```python
from build123d import *

# Parameters (mm, degrees)
BOSS_EXTRUDE1_DEPTH                = 25.4
FILLET1_R                          = 25.4
F_1_4_0_25_DIAMETER_SLOT1_DEPTH    = 25.4
F_1_16_0_0625_DIAMETER_HOLE1_D     = 1.5875
F_1_16_0_0625_DIAMETER_HOLE1_DEPTH = 12.7
F_1_16_0_0625_DIAMETER_HOLE1_TIP   = 0.476933116


# Read off the part's stored shape, not the designer's step: 1/4 (0.25) Diameter Slot1
with BuildPart() as part:
    # Sketch1 → Boss-Extrude1 (new body)
    with BuildSketch(Plane.XY):
        Polygon((-152.4, 0), (152.4, 0), (122.789463707, -63.5), (-122.789463707, -63.5), align=None)
    extrude(amount=BOSS_EXTRUDE1_DEPTH)

    # Fillet1
    fillet1_edges = [part.edges().sort_by_distance(p)[0] for p in [
        (122.789463707, -63.5, 12.7),
        (-122.789463707, -63.5, 12.7),
    ]]
    fillet(fillet1_edges, radius=FILLET1_R)

    # 1/4 (0.25) Diameter Slot1 outline → 1/4 (0.25) Diameter Slot1 (cut)
    with BuildSketch(Plane.XY):
        with BuildLine():
            Line((-92.075, -41.275), (92.075, -41.275))
            ThreePointArc((92.075, -41.275), (95.25, -38.1), (92.075, -34.925))
            Line((92.075, -34.925), (-92.075, -34.925))
            ThreePointArc((-92.075, -34.925), (-95.25, -38.1), (-92.075, -41.275))
        make_face()
    extrude(amount=F_1_4_0_25_DIAMETER_SLOT1_DEPTH, mode=Mode.SUBTRACT)

    # 1/16 (0.0625) Diameter Hole1
    with Locations(Plane(origin=(0, 0, 0), x_dir=(1, 0, 0), z_dir=(0, 1, 0))):
        with Locations((-101.6, -12.7), (-50.8, -12.7), (0, -12.7), (50.8, -12.7), (101.6, -12.7)):
            Hole(F_1_16_0_0625_DIAMETER_HOLE1_D / 2, depth=F_1_16_0_0625_DIAMETER_HOLE1_DEPTH)
            with Locations((0, 0, -(F_1_16_0_0625_DIAMETER_HOLE1_DEPTH + F_1_16_0_0625_DIAMETER_HOLE1_TIP / 2))):  # 118° drill point
                Cone(0, F_1_16_0_0625_DIAMETER_HOLE1_D / 2, F_1_16_0_0625_DIAMETER_HOLE1_TIP, mode=Mode.SUBTRACT)


solid = part.part
```
The listing builds one solid part. Answer for the finished solid, in the listing's coordinates (mm). A direction names the side the tool comes from. Coordinates: 2 decimals unless noted, no trailing zeros. Write each loop counter-clockwise with the first axis right and the second up, starting at its lowest first coordinate (ties: lowest second). Pieces come first, ordered by that corner, then holes. Notation, with made-up numbers: (26.5, 4) - (30.5, 4) arc R17 ccw to (30.5, 32) - close; hole circle Ø11 at (39, -23). An arc over 180 degrees is marked (long way). Return JSON: item names as keys, results as strings. Group by question number.
1. A cutting plane is placed at D-D, the plane y = -9.5. Determine the outline of the cut face in (x, z), plus the area to 3 significant figures.
2. Which of the six approach directions +Z, -Z, +X, -X, +Y, -Y give full straight-line access (tool end or side, diameter ignored) to faces 1 (the flat face through (1, -34.925, 13)), 2 (the flat face through (1, -63.5, 13))?
3. A cutting plane is placed at B-B, the plane y = -38.1. Determine the outline of the cut face in (x, z), plus the area to 3 significant figures.
4. Determine the mould class of faces 3 (the cylindrical face through (95.25, -38.17, 12.52)), 4 (the flat face through (2, -31, 0)), 5 (the cylindrical face through (120.425, -59.413, 12.878)), 6 (the flat face through (-1, -41.275, 13)) for opening direction X: released by +X, released by -X, zero draft, split by the parting line, or undercut.
5. A cutting plane is placed at A-A, the plane x = 82. Determine the outline of the cut face in (y, z) (3 decimals), plus the area to 3 significant figures.
6. Given pin 1 (4 mm diameter, centred on y = -37, z = 9.5, fed in from -X); pin 2 (1.4 mm diameter, centred on x = -50.8, z = 12.7, fed in from +Y); pin 3 (5 mm diameter, centred on y = -11, z = 22, fed in from -X), each flat-ended and moving along its own axis, determine where each tip first touches the part or whether it passes through.
7. Straight lines are drawn through the part: L1, parallel to Y at x = 20, z = 19.75 (3 decimals); L2, parallel to X at y = -7.25, z = 12.7; L3, parallel to X at y = -4.5, z = 12.7. For each, find the intervals that lie inside material, in ascending order.
Ans:
{
 "1": {"outline": "(-147.97, 0) - (147.97, 0) - (147.97, 25.4) - (-147.97, 25.4) - close; hole circle Ø1.59 at (-101.6, 12.7); hole circle Ø1.59 at (-50.8, 12.7); hole circle Ø1.59 at (0, 12.7); hole circle Ø1.59 at (50.8, 12.7); hole circle Ø1.59 at (101.6, 12.7)", "area": "7,510 mm²"},
 "2": {"face 1": "+Z, -Z", "face 2": "+Z, -Z, +X, -X, -Y"},
 "3": {"outline": "(-134.63, 0) - (-95.25, 0) - (-95.25, 25.4) - (-134.63, 25.4) - close; (95.25, 0) - (134.63, 0) - (134.63, 25.4) - (95.25, 25.4) - close", "area": "2,000 mm²"},
 "4": {"face 3": "undercut", "face 4": "zero draft", "face 5": "released by +X", "face 6": "undercut"},
 "5": {"outline": "(-63.5, 0) - (-41.275, 0) - (-41.275, 25.4) - (-63.5, 25.4) - close; (-34.925, 0) - (0, 0) - (0, 25.4) - (-34.925, 25.4) - close", "area": "1,450 mm²"},
 "6": {"pin 1": "x = -136.08", "pin 2": "y = -12.76", "pin 3": "x = -148.44"},
 "7": {"L1": "-63.5 to -41.275, -34.925 to 0", "L2": "-149.02 to -102.39, -100.81 to -51.59, -50.01 to -0.79, 0.79 to 50.01, 51.59 to 100.81, 102.39 to 149.02", "L3": "-150.3 to -102.39, -100.81 to -51.59, -50.01 to -0.79, 0.79 to 50.01, 51.59 to 100.81, 102.39 to 150.3"}
}
